from build123d import *

# Parameters (mm, degrees)
F1_DEPTH = 9.525


with BuildPart() as f1:
    # F0 (on Top) → F1 (new body)
    with BuildSketch(Plane.XY):
        with BuildLine():
            Line((25.4, -37.084), (25.4, 82.55))
            Line((25.4, 82.55), (-25.4, 82.55))
            Line((-25.4, 82.55), (-25.4, -37.084))
            Line((-25.4, -37.084), (-21.353429, -41.388863))
            ThreePointArc((-21.353429, -41.388863), (-18.800003, -45.409099), (-17.907, -50.08722))
            Line((-17.907, -50.08722), (-17.907, -63.5))
            Line((-17.907, -63.5), (0, -82.55))
            Line((0, -82.55), (17.907, -63.5))
            Line((17.907, -63.5), (17.907, -50.08722))
            ThreePointArc((17.907, -50.08722), (18.800003, -45.409099), (21.353429, -41.388863))
            Line((21.353429, -41.388863), (25.4, -37.084))
        make_face()
        with BuildLine():
            ThreePointArc((1.5875, 63.5), (6.35, 68.2625), (11.1125, 63.5))
            Line((11.1125, 63.5), (11.1125, 44.45))
            ThreePointArc((11.1125, 44.45), (6.35, 39.6875), (1.5875, 44.45))
            Line((1.5875, 44.45), (1.5875, 63.5))
        make_face(mode=Mode.SUBTRACT)
    extrude(amount=F1_DEPTH)


solid = f1.part
Work out the finished part from the listing and answer in its coordinate system (mm). A direction names the side the tool comes from. Give positions to 0.01 mm unless a question says otherwise; leave off trailing zeros. Order: outer loops, then holes, each group sorted by start corner. A loop starts at its lowest first (then second) coordinate and runs counter-clockwise, first axis right, second up. Notation, with made-up numbers: (14, -22.75) -> (55, -22.75) arc R26 cw to (55, -5.75) -> close; hole circle Ø3 at (9.25, 76.5). An arc over 180 degrees is marked (long way). One line per item, written item: value.
Item 1: Determine the mould class of faces 5 (the flat face through (-23.405, -39.206, 4.696)), 6 (the flat face through (0, 1, 0)), 7 (the flat face through (11.112, 54, 5)) for opening direction Y: released by +Y, released by -Y, zero draft, split by the parting line, or undercut.
Answer sheet:
face 5: released by -Y
face 6: zero draft
face 7: undercut
Item 2: Straight lines are drawn through the part: probe 1 along X at (y, z) = (-49.5, 9); probe 2 along X at (y, z) = (-73, 2); probe 3 along X at (y, z) = (42.5, 6.5). For each, find the intervals that lie inside material, in ascending order.
Answer sheet:
probe 1: -17.92 to 17.92
probe 2: -8.98 to 8.98
probe 3: -25.4 to 2.01, 10.69 to 25.4
Item 3: A tool of negligible diameter and unlimited length cuts with its end or side. For faces 1 (the flat face through (-17.907, -57, 5)), 2 (the flat face through (0, 1, 9.525)), 3 (the flat face through (17.907, -57, 5)), 4 (the cylindrical face through (6.45, 39.69, 4.7)), from which of +Z, -Z, +X, -X, +Y, -Y can it reach the whole face along a straight path? Write none if from no direction.
Answer sheet:
face 1: +Z, -Z, -X, -Y
face 2: +Z, +X, -X, +Y, -Y
face 3: +Z, -Z, +X, -Y
face 4: +Z, -Z
Item 4: Find section B-B, the plane x = 3. Give the vertices of the cut face in (y, z) (3 decimals).
Answer sheet:
outline: (-79.359, 0) -> (41.065, 0) -> (41.065, 9.525) -> (-79.359, 9.525) -> close; (66.885, 0) -> (82.55, 0) -> (82.55, 9.525) -> (66.885, 9.525) -> close
